```python
from build123d import *

# Parameters (mm, degrees)
F1_DEPTH = 1.524
F3_DEPTH = 1.524
F6_D     = 3.175


with BuildPart() as f1:
    # F0 (on Front) → F1 (new body)
    with BuildSketch(Plane.XZ):
        with BuildLine():
            Line((6.35, 17.78), (-6.35, 17.78))
            Line((-6.35, 17.78), (-6.35, -11.43))
            ThreePointArc((-6.35, -11.43), (-4.4901280605, -15.9201280605), (0, -17.78))
            ThreePointArc((0, -17.78), (4.4901280605, -15.9201280605), (6.35, -11.43))
            Line((6.35, -11.43), (6.35, 17.78))
        make_face()
    extrude(amount=F1_DEPTH)

    # F2 (on face) → F3 (join)
    with BuildSketch(Plane.YZ.offset(6.35)):
        with BuildLine():
            add(Edge.make_bspline(
                [(0, -6.5310765533), (2.3925540429, -1.2585692564), (2.3925540429, -2.2239157952), (7.2943206633, 0)],
                knots=[0, 0, 0, 0, 9.7909179796, 9.7909179796, 9.7909179796, 9.7909179796], degree=3))
            ThreePointArc((7.2943206633, 0), (10.16, 4.572), (7.2943206633, 9.144))
            add(Edge.make_bspline(
                [(0, 15.6750765533), (2.3925540429, 10.4025692564), (2.3925540429, 11.3679157952), (7.2943206633, 9.144)],
                knots=[0, 0, 0, 0, 9.7909179796, 9.7909179796, 9.7909179796, 9.7909179796], degree=3))
            Line((0, 15.6750765533), (0, -6.5310765533))
        make_face()
    extrude(amount=-F3_DEPTH)

    # F4: F1 across plane


with BuildPart() as f1_1:
    add(f1.part)
    add(f1.part.mirror(Plane.YZ))

    # F6 (through all)
    with Locations(Plane.YZ.offset(6.35)):
        with Locations((5.08, 4.572)):
            Hole(F6_D / 2)


solid = f1_1.part
```
For this review, take the finished solid that the model builds, in its own axes (mm). A direction names the side the tool comes from. Round coordinates to 2 decimals unless told otherwise and drop trailing zeros. Write each loop counter-clockwise with the first axis right and the second up, starting at its lowest first coordinate (ties: lowest second). Pieces come first, ordered by that corner, then holes. Notation, with made-up numbers: (46, 39.25) -> (100, 39.25) arc R25 ccw to (100, 75.25) -> close; hole circle Ø5 at (6.25, 44). An arc over 180 degrees is marked (long way). One line per question, with ' | ' between items. Start each with the question number.
(1) Mouldability with a two-part tool opening along X and no side actions: class faces 1 (the face through (-6.35, 3, 3)), 2 (the face through (5.6, 10.16, 4.49)), 3 (the face through (0, 0, 0)) as released by +X, released by -X, zero draft, split by the parting line, or undercut.
(2) Add section D-D, the plane x = -1.5. Write out the cut boundary in (y, z), plus the area to 3 significant figures.
(3) Insertion check: P1, Ø6, axis at x = -2.5, z = -9, coming from the +Y side. The pin has a flat end and moves straight along its axis. Give the tip position at first contact, or say it passes through.
(4) Add section C-C, the plane y = 5.5. Give the number of separate pieces and of enclosed holes in the cut face, plus the area to 3 significant figures.
(5) Tool access review of faces 4 (the face through (-4.826, 3, 5)), 5 (the face through (5.577, 4.347, 3.164)): name each direction out of +Z, -Z, +X, -X, +Y, -Y from which nothing blocks a thin tool from reaching the whole face with its end or side.
(6) For line 1 along X through (y, z) = (3.25, 6); line 2 along Y through (x, z) = (0.25, 9); line 3 along Z through (x, y) = (5.5, 8.5), list the stretches that pass through material, from the lowest coordinate up. Write a range as from..to.
(7) Add section B-B, the plane z = -10. Write out the cut boundary in (x, y).
(8) Add section A-A, the plane z = 4. Write out the cut boundary in (x, y), plus the area to 3 significant figures.
Answer list:
1) face 1: released by -X | face 2: zero draft | face 3: undercut
2) outline: (-1.52, -17.6) -> (0, -17.6) -> (0, 17.78) -> (-1.52, 17.78) -> close | area: 53.9 mm²
3) P1: y = 0
4) separate pieces: 4 | enclosed holes: 0 | area: 23.3 mm²
5) face 4: +Z, -Z, +Y | face 5: +X, -X
6) line 1: -6.35..-4.83, 4.83..6.35 | line 2: -1.52..0 | line 3: 0.82..8.33
7) outline: (-6.35, -1.52) -> (6.35, -1.52) -> (6.35, 0) -> (-6.35, 0) -> close
8) outline: (-6.35, -1.52) -> (6.35, -1.52) -> (6.35, 3.6) -> (4.83, 3.6) -> (4.83, 0) -> (-4.83, 0) -> (-4.83, 3.6) -> (-6.35, 3.6) -> close; (-6.35, 6.56) -> (-4.83, 6.56) -> (-4.83, 10.13) -> (-6.35, 10.13) -> close; (4.83, 6.56) -> (6.35, 6.56) -> (6.35, 10.13) -> (4.83, 10.13) -> close | area: 41.2 mm²
